from build123d import *

# Parameters (mm, degrees)
F0_W     = 90
F0_H     = 20
F1_DEPTH = 5
F2_T     = -2.5
F4_D     = 6.2


with BuildPart() as f1:
    # F0 (on Front) → F1 (new body)
    with BuildSketch(Plane.XZ):
        Rectangle(F0_W, F0_H)
    extrude(amount=F1_DEPTH)

    # F2
    f2_openings = [f1.faces().sort_by_distance(p)[0] for p in [
        (0, 0, 0),
        (45, -2.5, 0),
        (-45, -2.5, 0),
    ]]
    offset(amount=F2_T, openings=f2_openings)

    # F4 (through all)
    with Locations(Plane.XZ.offset(5)):
        with Locations((40, 0), (-40, 0)):
            Hole(F4_D / 2)


solid = f1.part
The model under review builds one solid part; all positions refer to its coordinate system, in mm. A direction names the side the tool comes from. Coordinates: 2 decimals unless noted, no trailing zeros. Write each loop counter-clockwise with the first axis right and the second up, starting at its lowest first coordinate (ties: lowest second). Pieces come first, ordered by that corner, then holes. Notation, with made-up numbers: (26, 82.5) - (39, 82.5) arc R25 cw to (39, 107.5) - close; hole circle Ø7 at (69.5, 63.25). An arc over 180 degrees is marked (long way). Answer as a JSON object with one key per item and string values. Group by question number.
1. To check wall thickness, follow probe 1 along X at (y, z) = (-4.3, -0.25); probe 2 along Z at (x, y) = (4, -0.75); probe 3 along Z at (x, y) = (40, -4.25). State the ranges of each line that lie inside material, in increasing order.
2. Add section A-A (z = 0). Give the boundary of the cut face in (x, y).
3. Mouldability with a two-part tool opening along X and no side actions: class faces 1 (the face through (45, -4, 0)), 2 (the face through (37.136, -3.733, -1.187)), 3 (the face through (-1, -1, -7.5)), 4 (the face through (-45, -4, 0)) as pulls with the +X half, pulls with the -X half, needs draft (parallel to the pull), parting line crosses it, or undercut.
4. Add section B-B (x = -40). Give the boundary of the cut face in (y, z), plus the area to 3 significant figures.
5. Add section D-D (z = -6). Give the boundary of the cut face in (x, y), plus the area to 3 significant figures.
6. Add section C-C (y = -4.1). Give the boundary of the cut face in (x, z), plus the area to 3 significant figures.
7. Clearance check with flat-ended pins moving along their axes: pin 1 Ø5 at (x, z) = (27, 2.5) entering from +Y; pin 2 Ø10 at (x, z) = (-0.5, -7.5) entering from +Y. State where each tip first meets the part, or that it passes through.
8. Machinability: for faces 5 (the face through (-1, -2, 10)), 6 (the face through (-1, -2.5, 0)), which of the approach directions +Z, -Z, +X, -X, +Y, -Y give a long, thin tool a straight path to every point of the face, cutting with its end or side? Answer none if there is none.
Findings:
{
 "1": {"probe 1": "-45 to -43.09, -36.91 to 36.91, 43.09 to 45", "probe 2": "-10 to -7.5, 7.5 to 10", "probe 3": "-10 to -3.1, 3.1 to 10"},
 "2": {"outline": "(-45, -5) - (-43.1, -5) - (-43.1, -2.5) - (-45, -2.5) - close; (-36.9, -5) - (36.9, -5) - (36.9, -2.5) - (-36.9, -2.5) - close; (43.1, -5) - (45, -5) - (45, -2.5) - (43.1, -2.5) - close"},
 "3": {"face 1": "pulls with the +X half", "face 2": "undercut", "face 3": "needs draft", "face 4": "pulls with the -X half"},
 "4": {"outline": "(-5, -10) - (0, -10) - (0, -7.5) - (-2.5, -7.5) - (-2.5, -3.1) - (-5, -3.1) - close; (-5, 3.1) - (-2.5, 3.1) - (-2.5, 7.5) - (0, 7.5) - (0, 10) - (-5, 10) - close", "area": "47.0 mm²"},
 "5": {"outline": "(-45, -5) - (45, -5) - (45, -2.5) - (-45, -2.5) - close", "area": "225 mm²"},
 "6": {"outline": "(-45, -10) - (45, -10) - (45, 10) - (-45, 10) - close; hole circle Ø6.2 at (-40, 0); hole circle Ø6.2 at (40, 0)", "area": "1,740 mm²"},
 "7": {"pin 1": "y = -2.5", "pin 2": "y = 0"},
 "8": {"face 5": "+Z, +X, -X, +Y, -Y", "face 6": "+X, -X, +Y"}
}
